Could you check a few things on this drawing? It's one solid part, dimensions in mm from its lowest x, y, z. Give positions to 0.01 mm unless a question says otherwise; leave off trailing zeros. Loops run counter-clockwise (first coordinate to the right, second up) from the corner with the lowest first, then second, coordinate; pieces in that order, holes last.
1. Imagine slicing it at D-D (z = 0.5). List the corners of the cut face in (x, y) for me (1 decimal).
2. Imagine slicing it at C-C (y = 41). List the corners of the cut face in (x, z) for me (1 decimal), plus the area to 3 significant figures.
3. Imagine slicing it at B-B (x = 13.3). List the corners of the cut face in (y, z) for me.
4. Thinking about a two-plate mould opening in Y: for the marked faces 1, 2 and 3, which applies, +Y half, -Y half, draft (parallel to the pull), parting line (faces both ways), or undercut?
5. For P1, Ø3, axis at x = 13.5, z = 1, coming from the -Y side; P2, Ø4, axis at x = 13.3, y = 39.85, coming from the -Z side; P3, Ø1.5, axis at x = 22.8, y = 2.5, coming from the -Z side, each with a flat end and sliding along its axis, tell me the tip position at first contact or that it passes through.
6. Imagine slicing it at A-A (y = 2.5). List the corners of the cut face in (x, z) for me, plus the area to 3 significant figures.
7. I need wall thicknesses on line 1 along X through (y, z) = (22.5, 5.95); line 2 along X through (y, z) = (23, 4); line 3 along Z through (x, y) = (5.75, 31). Which ranges of each line are inside material? Lowest first, please.
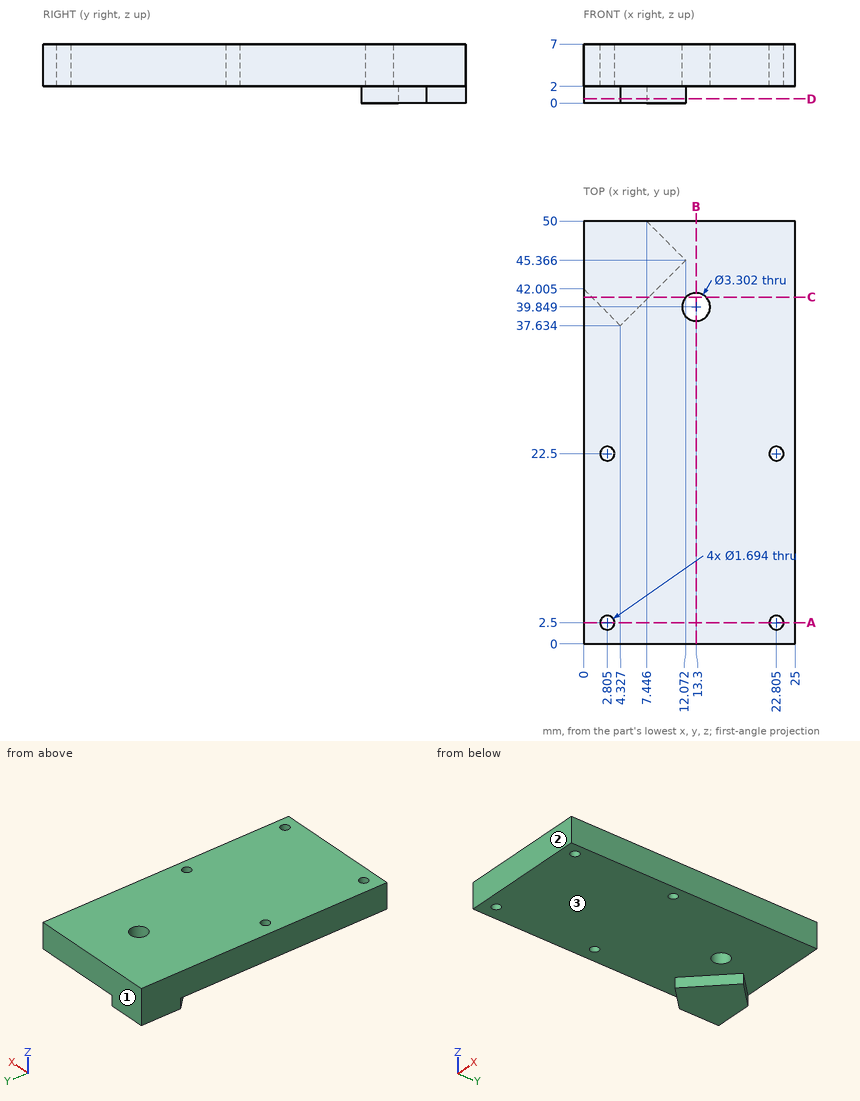
Derived:
1. outline: (0, 42) - (4.3, 37.6) - (12.1, 45.4) - (7.4, 50) - (0, 50) - close
2. outline: (0, 2) - (1, 2) - (1, 0) - (7.7, 0) - (7.7, 2) - (12.1, 2) - (12.1, 7) - (0, 7) - close; (14.5, 2) - (25, 2) - (25, 7) - (14.5, 7) - close
2. area: 127 mm2
3. outline: (0, 2) - (38.2, 2) - (38.2, 7) - (0, 7) - close; (41.5, 2) - (50, 2) - (50, 7) - (41.5, 7) - close
4. face 1: +Y half
4. face 2: -Y half
4. face 3: draft
5. P1: stops at y = 0
5. P2: stops at z = 2
5. P3: passes through
6. outline: (0, 2) - (1.96, 2) - (1.96, 7) - (0, 7) - close; (3.65, 2) - (21.96, 2) - (21.96, 7) - (3.65, 7) - close; (23.65, 2) - (25, 2) - (25, 7) - (23.65, 7) - close
6. area: 108 mm2
7. line 1: x = 0 to 1.96, 3.65 to 21.96, 23.65 to 25
7. line 2: x = 0 to 2.12, 3.49 to 22.12, 23.49 to 25
7. line 3: z = 2 to 7
